Design review of the part built by this model. Coordinates are the model's own, in mm. Coordinates: 2 decimals unless noted, no trailing zeros. One line per question, with ' | ' between items. Start each with the question number.
Q1. For P1, Ø5, axis at x = -0.5, y = 1, coming from the -Z side; P2, Ø4, axis at x = -4.5, z = 9.5, coming from the -Y side; P3, Ø4, axis at y = 1.5, z = 10, coming from the -X side; P4, Ø1.3, axis at x = 0, y = 0, coming from the -Z side, all flat-tipped, find the tip position at first contact; note any pin that passes through.
Q2. Wall thickness on probe 1 along Y at (x, z) = (0, 3.4); probe 2 along X at (y, z) = (-1, -2); probe 3 along Y at (x, z) = (0.5, 1.75): over which ranges is each line inside the solid? List them lowest first.
Q3. Draft analysis for pull direction Y (two halves, no side actions). For faces 1 (the conical face through (-1.911, -3.674, 2.726)), 2 (the conical face through (0.366, -1.649, 8.653)), 3 (the flat face through (5, 3, -2.399)), state which applies: pulls with the +Y half, pulls with the -Y half, needs draft (parallel to the pull), parting line crosses it, or undercut.
from build123d import *


with BuildPart() as f1:
    # F0 (on Front) → F1 (revolve)
    with BuildSketch(Plane.XZ):
        with BuildLine():
            Line((-0.811438, 6.137778), (-3.027734, 12.491356))
            ThreePointArc((-3.027734, 12.491356), (-5.014969, 8.704305), (-3.347156, 4.766126))
            Line((-3.347156, 4.766126), (-6.137301, -2.39948))
            Line((-6.137301, -2.39948), (-5.197422, -2.39948))
            ThreePointArc((-5.197422, -2.39948), (-3.947176, 0.822017), (-0.953815, 2.548559))
            Line((-0.953815, 2.548559), (-0.811438, 2.733914))
            Line((-0.811438, 2.733914), (-0.811438, 6.137778))
        make_face()
    revolve(axis=Axis((0, 0, 4.58246), (0, 0, -1)))


solid = f1.part
Output values:
1) P1: stops at z = 1.17 | P2: stops at y = -4.29 | P3: stops at x = -5.02 | P4: passes through
2) probe 1: y = -3.88 to -0.81, 0.81 to 3.88 | probe 2: x = -5.9 to -5.07, 5.07 to 5.9 | probe 3: y = -4.49 to -2.86, 2.86 to 4.49
3) face 1: parting line crosses it | face 2: undercut | face 3: needs draft
